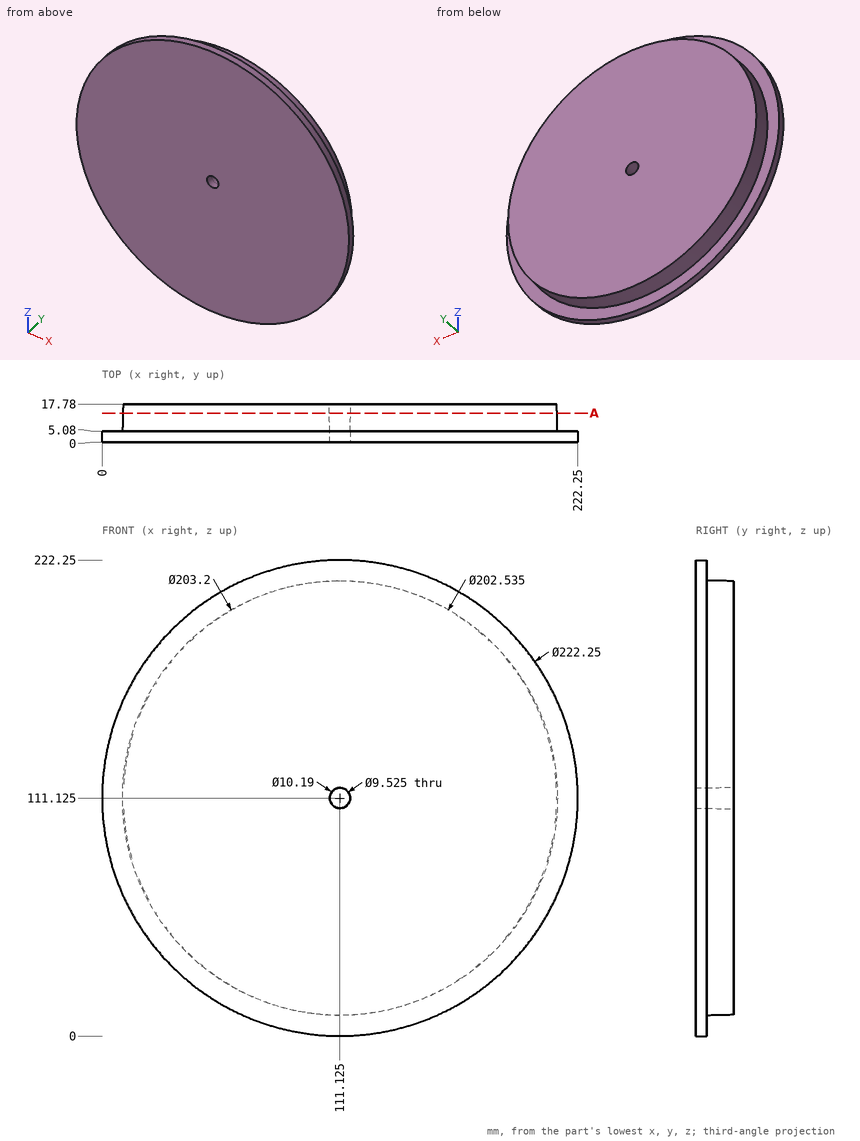
For this review, use the dimensioned drawing (mm, ordinates from the lowest corner) and the shaded views. Round coordinates to 2 decimals unless told otherwise and drop trailing zeros. Order: outer loops, then holes, each group sorted by start corner. A loop starts at its lowest first (then second) coordinate and runs counter-clockwise, first axis right, second up.
1) For L1, parallel to X at y = 3.5, z = 109; L2, parallel to Z at x = 104, y = 7.5; L3, parallel to X at y = 6, z = 72, list the stretches that pass through material, from the lowest coordinate up.
The answers:
L1: x = 0.02 to 106.86, 115.39 to 222.23
L2: z = 9.84 to 212.41
L3: x = 17.39 to 204.86
2) Consider section A-A (y = 13.5). State the section outline as (x, z) points (1 decimal), plus the area to 3 significant figures.
The answers:
outline: circle Ø202.8 at (111.1, 111.1); hole circle Ø10 at (111.1, 111.1)
area: 32,200 mm2
3) Clearance check with flat-ended pins moving along their axes: pin 1 Ø5 at (y, z) = (9, 40) entering from -X; pin 2 Ø2 at (x, y) = (184, 13) entering from +Z; pin 3 Ø1.5 at (y, z) = (5.5, 156.5) entering from -X; pin 4 Ø8.5 at (x, z) = (111.125, 111.125) entering from -Y. State where each tip first meets the part, or that it passes through.
The answers:
pin 1: stops at x = 36.34
pin 2: stops at z = 182.64
pin 3: stops at x = 9.41
pin 4: passes through
